Part model, mm, in its own coordinate system. A direction names the side the tool comes from. Round coordinates to 2 decimals unless told otherwise and drop trailing zeros. Order: outer loops, then holes, each group sorted by start corner. A loop starts at its lowest first (then second) coordinate and runs counter-clockwise, first axis right, second up. Notation, with made-up numbers: (15, -17) - (60, -17) arc R20 ccw to (60, 11) - close; hole circle Ø9 at (50, -23). An arc over 180 degrees is marked (long way). Answer as a JSON object with one key per item and string values.
```python
from build123d import *

# Parameters (mm, degrees)
SKETCH1_W           = 9.6
SKETCH1_H           = 11.3
BOSS_EXTRUDE1_DEPTH = 7
SKETCH2_R           = 3.35
BOSS_EXTRUDE2_DEPTH = 5
SKETCH3_R           = 2.3
BOSS_EXTRUDE3_DEPTH = 4
FILLET1_R           = 1
SKETCH4_R           = 2.9
BOSS_EXTRUDE4_DEPTH = 5.7


with BuildPart() as part:
    # Sketch1 → Boss-Extrude1 (new body)
    with BuildSketch(Plane(origin=(0, 0, 0), x_dir=(1, 0, 0), z_dir=(0, 1, 0))):
        Rectangle(SKETCH1_W, SKETCH1_H)
    extrude(amount=BOSS_EXTRUDE1_DEPTH)

    # Sketch2 → Boss-Extrude2 (add)
    with BuildSketch(Plane(origin=(0, 7, 0), x_dir=(1, 0, 0), z_dir=(0, 1, 0))):
        Circle(SKETCH2_R)
    extrude(amount=BOSS_EXTRUDE2_DEPTH)

    # Sketch3 → Boss-Extrude3 (add)
    with BuildSketch(Plane(origin=(0, 12, 0), x_dir=(1, 0, 0), z_dir=(0, 1, 0))):
        Circle(SKETCH3_R)
    extrude(amount=BOSS_EXTRUDE3_DEPTH)

    # Fillet1
    fillet1_edges = [part.edges().sort_by_distance(p)[0] for p in [
        (-2.3, 12, 0),
    ]]
    fillet(fillet1_edges, radius=FILLET1_R)

    # Sketch4 → Boss-Extrude4 (add)
    with BuildSketch(Plane(origin=(0, 16, 0), x_dir=(1, 0, 0), z_dir=(0, 1, 0))):
        Circle(SKETCH4_R)
    extrude(amount=BOSS_EXTRUDE4_DEPTH)


solid = part.part
```
Item 1: Two-plate mould, pull along Y, no slides. Class faces 1 (the flat face through (-2, 7, -3)), 2 (the flat face through (0, 0, 0)), 3 (the cylindrical face through (-1.825, 14.479, 1.4)): pulls with the +Y half, pulls with the -Y half, needs draft (parallel to the pull), parting line crosses it, or undercut.
Taken from the geometry:
{"face 1": "pulls with the +Y half", "face 2": "pulls with the -Y half", "face 3": "undercut"}
Item 2: Cut at C-C (y = 7.25). Write the cut outline in (x, z).
Taken from the geometry:
{"outline": "circle Ø6.7 at (0, 0)"}
Item 3: Probe L1, parallel to Y at x = 0.75, z = -5; L2, parallel to X at y = 18.5, z = -1.25; L3, parallel to Z at x = -2, y = 15.5. List the from-to ranges inside material, lowest first. Write a range as from..to.
Taken from the geometry:
{"L1": "0..7", "L2": "-2.62..2.62", "L3": "-1.14..1.14"}
Item 4: Cut at D-D (x = -4). Write the cut outline in (y, z), plus the area to 3 significant figures.
Taken from the geometry:
{"outline": "(0, -5.65) - (7, -5.65) - (7, 5.65) - (0, 5.65) - close", "area": "79.1 mm2"}
Item 5: Tool access for faces 4 (the flat face through (-4.8, 3, 0)), 5 (the cylindrical face through (-2.9, 18.8, -0.1)): list every direction of +Z, -Z, +X, -X, +Y, -Y with a clear straight run to the whole face (end or side of a thin tool).
Taken from the geometry:
{"face 4": "+Z, -Z, -X, +Y, -Y", "face 5": "+Y"}
Item 6: Drop flat-ended pins along their axis: P1, Ø1.5, axis at x = 3, y = 17, coming from the -Z side; P2, Ø1, axis at x = -3.5, y = 8.5, coming from the -Z side; P3, Ø1, axis at y = 9.5, z = 0, coming from the -X side. Give the stop position or say it passes through.
Taken from the geometry:
{"P1": "z = -1.83", "P2": "z = -1.49", "P3": "x = -3.35"}
Item 7: Cut at A-A (z = 0). Write the cut outline in (x, y), plus the area to 3 significant figures.
Taken from the geometry:
{"outline": "(-4.8, 0) - (4.8, 0) - (4.8, 7) - (3.35, 7) - (3.35, 12) - (3.3, 12) arc R1 cw to (2.3, 13) - (2.3, 16) - (2.9, 16) - (2.9, 21.7) - (-2.9, 21.7) - (-2.9, 16) - (-2.3, 16) - (-2.3, 13) arc R1 cw to (-3.3, 12) - (-3.35, 12) - (-3.35, 7) - (-4.8, 7) - close", "area": "153 mm2"}
Item 8: Cut at B-B (x = 0). Write the cut outline in (y, z).
Taken from the geometry:
{"outline": "(0, -5.65) - (7, -5.65) - (7, -3.35) - (12, -3.35) - (12, -3.3) arc R1 cw to (13, -2.3) - (16, -2.3) - (16, -2.9) - (21.7, -2.9) - (21.7, 2.9) - (16, 2.9) - (16, 2.3) - (13, 2.3) arc R1 cw to (12, 3.3) - (12, 3.35) - (7, 3.35) - (7, 5.65) - (0, 5.65) - close"}
